```python
from build123d import *

# Parameters (mm, degrees)
F0_W     = 4.7515250481
F0_H     = 22.4042496848
F1_DEPTH = 4.445


with BuildPart() as f1:
    # F0 (on Front) → F1 (new body)
    with BuildSketch(Plane.XZ):
        with BuildLine():
            Line((-107.0503221856, -3.0948602284), (-76.2880815111, 0))
            Line((-76.2880815111, 0), (-86.7243445437, 103.7341952324))
            Line((-86.7243445437, 103.7341952324), (-53.7250275092, 57.9696269721))
            ThreePointArc((-53.7250275092, 57.9696269721), (-46.1566377564, 60.2633619864), (-38.773926276, 57.4283461196))
            Line((-38.773926276, 57.4283461196), (0, 103.7341952324))
            Line((0, 103.7341952324), (40.0807997492, 57.3092244379))
            ThreePointArc((40.0807997492, 57.3092244379), (47.3933296143, 60.2539299742), (54.9783525161, 58.1064171563))
            Line((54.9783525161, 58.1064171563), (86.548257701, 103.7341875683))
            Line((86.548257701, 103.7341875683), (76.1119184889, 0))
            Line((76.1119184889, 0), (106.8741568907, -3.0948828193))
            Line((106.8741568907, -3.0948828193), (148.2956194489, 138.5004273575))
            Line((148.2956194489, 138.5004273575), (-148.4725865748, 138.5004273575))
            Line((-148.4725865748, 138.5004273575), (-107.0503221856, -3.0948602284))
        make_face()
        Polygon((-45.5729805496, 127.6698307823), (-45.5729805496, 109.2178300023), (-50.3245055976, 109.2178300023), (-50.3245055976, 127.6698307823), (-56.4097920627, 127.6698307823), (-56.4097920627, 131.6220796871), (-39.4925976191, 131.6220796871), (-39.4925976191, 127.6698307823), align=None, mode=Mode.SUBTRACT)
        with Locations((-33.6696502563, 120.4199548447)):
            Rectangle(F0_W, F0_H, mode=Mode.SUBTRACT)
        Polygon((-11.0520968155, 113.1406576994), (-11.0520968155, 109.2178300023), (-27.724114528, 109.2178300023), (-27.724114528, 112.2972497445), (-16.9804701727, 127.69925199), (-27.4299024507, 127.69925199), (-27.4299024507, 131.6220796871), (-11.3414053582, 131.6220796871), (-11.3414053582, 128.5573705488), (-22.0703391096, 113.1406576994), align=None, mode=Mode.SUBTRACT)
        Polygon((7.120402491, 113.1406576994), (7.120402491, 109.2178300023), (-9.5516152214, 109.2178300023), (-9.5516152214, 112.2972497445), (1.1920291339, 127.69925199), (-9.2574031441, 127.69925199), (-9.2574031441, 131.6220796871), (6.8310939484, 131.6220796871), (6.8310939484, 128.5573705488), (-3.8978398031, 113.1406576994), align=None, mode=Mode.SUBTRACT)
        with Locations((13.0659382194, 120.4199548447)):
            Rectangle(F0_W, F0_H, mode=Mode.SUBTRACT)
        Polygon((34.9185402592, 109.2178300023), (21.0807655579, 109.2178300023), (21.0807655579, 131.6220796871), (25.832290606, 131.6220796871), (25.832290606, 113.1406576994), (34.9185402592, 113.1406576994), align=None, mode=Mode.SUBTRACT)
        Polygon((41.1411256937, 131.6220796871), (45.7847729801, 122.3985310644), (50.4578414742, 131.6220796871), (55.5771316188, 131.6220796871), (48.1433731329, 117.936314559), (48.1433731329, 109.2178300023), (43.4261728272, 109.2178300023), (43.4261728272, 117.7843049857), (35.9924143413, 131.6220796871), align=None, mode=Mode.SUBTRACT)
        with BuildLine():
            Line((-46.5975366533, 48.0849817395), (-53.7250275092, 57.9696269721))
            ThreePointArc((-53.7250275092, 57.9696269721), (-52.1495262693, 37.2368137569), (-34.411177998, 48.0849817395))
            Line((-34.411177998, 48.0849817395), (-46.5975366533, 48.0849817395))
        make_face()
        with BuildLine():
            ThreePointArc((-38.773926276, 57.4283461196), (-46.1566377564, 60.2633619864), (-53.7250275092, 57.9696269721))
            Line((-53.7250275092, 57.9696269721), (-46.5975366533, 48.0849817395))
            Line((-46.5975366533, 48.0849817395), (-38.773926276, 57.4283461196))
        make_face()
        with BuildLine():
            Line((-38.773926276, 57.4283461196), (-46.5975366533, 48.0849817395))
            Line((-46.5975366533, 48.0849817395), (-34.411177998, 48.0849817395))
            ThreePointArc((-34.411177998, 48.0849817395), (-35.555601603, 53.240852919), (-38.773926276, 57.4283461196))
        make_face()
        with BuildLine():
            ThreePointArc((60.230868841, 48.0849817395), (58.838157085, 53.7422358339), (54.9783525161, 58.1064171563))
            Line((54.9783525161, 58.1064171563), (48.0445101857, 48.0849817395))
            Line((48.0445101857, 48.0849817395), (35.8581515305, 48.0849817395))
            ThreePointArc((35.8581515305, 48.0849817395), (48.0445101857, 35.8986230843), (60.230868841, 48.0849817395))
        make_face()
        with BuildLine():
            Line((48.0445101857, 48.0849817395), (54.9783525161, 58.1064171563))
            ThreePointArc((54.9783525161, 58.1064171563), (47.3933296143, 60.2539299742), (40.0807997492, 57.3092244379))
            Line((40.0807997492, 57.3092244379), (48.0445101857, 48.0849817395))
        make_face()
        with BuildLine():
            Line((48.0445101857, 48.0849817395), (40.0807997492, 57.3092244379))
            ThreePointArc((40.0807997492, 57.3092244379), (36.9639874345, 53.1573926884), (35.8581515305, 48.0849817395))
            Line((35.8581515305, 48.0849817395), (48.0445101857, 48.0849817395))
        make_face()
    extrude(amount=F1_DEPTH)


solid = f1.part
```
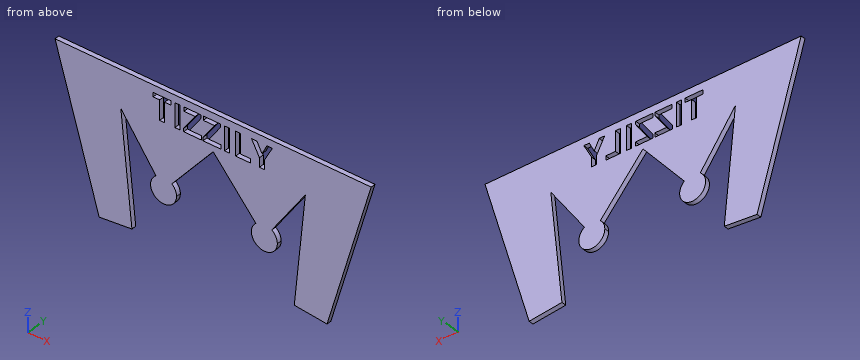
Source: CAD feature listing. Evaluate the final solid. Frame: model axes, mm. Coordinates: 2 decimals unless noted, no trailing zeros. Write each loop counter-clockwise with the first axis right and the second up, starting at its lowest first coordinate (ties: lowest second). Pieces come first, ordered by that corner, then holes. Notation, with made-up numbers: (-24.75, -37.5) - (16.25, -37.5) arc R25 cw to (16.25, -10.5) - close; hole circle Ø2 at (11.25, 78). An arc over 180 degrees is marked (long way). Answer as a JSON object with one key per item and string values.
Q1. Section query B-B, the plane y = -3.05. State how many separate pieces and enclosed holes the cut face has, plus the area to 3 significant figures.
Ans:
{"separate pieces": "1", "enclosed holes": "7", "area": "23,200 mm2"}
Q2. Section query A-A, the plane z = 69.5. Output: boundary loops of the cut face in (x, y) (3 decimals).
Ans:
{"outline": "(-128.287, -4.445) - (-83.28, -4.445) - (-83.28, 0) - (-128.287, 0) - close; (-62.039, -4.445) - (-28.666, -4.445) - (-28.666, 0) - (-62.039, 0) - close; (29.556, -4.445) - (62.862, -4.445) - (62.862, 0) - (29.556, 0) - close; (83.104, -4.445) - (128.111, -4.445) - (128.111, 0) - (83.104, 0) - close"}
Q3. First-contact query: pin 1 Ø2 at (y, z) = (-1.5, 123.5) entering from +X; pin 2 Ø1.2 at (y, z) = (-2.5, 112) entering from -X; pin 3 Ø2 at (x, y) = (-35, -1.5) entering from -Z. Flat tips, straight axial feed; report the tip coordinate or a pass-through.
Ans:
{"pin 1": "stops at x = 144.2", "pin 2": "stops at x = -140.9", "pin 3": "stops at z = 42.07"}
Q4. Section query C-C, the plane z = 41. Output: boundary loops of the cut face in (x, y) (3 decimals).
Ans:
{"outline": "(-119.95, -4.445) - (-80.413, -4.445) - (-80.413, 0) - (-119.95, 0) - close; (-56.513, -4.445) - (-36.682, -4.445) - (-36.682, 0) - (-56.513, 0) - close; (38.129, -4.445) - (57.96, -4.445) - (57.96, 0) - (38.129, 0) - close; (80.237, -4.445) - (119.773, -4.445) - (119.773, 0) - (80.237, 0) - close"}
Q5. Material intervals for line 1 (X direction, y = -0.7, z = 37.5); line 2 (Z direction, x = -12, y = -2.9); line 3 (X direction, y = -1.85, z = 70), sorted ascending. Write a range as [from, to].
Ans:
{"line 1": "x = [-118.93, -80.06], [-52.64, -40.56], [42.01, 54.08], [79.88, 118.75]", "line 2": "z = [89.4, 109.22], [113.14, 127.61], [131.62, 138.5]", "line 3": "x = [-128.43, -83.33], [-62.4, -28.25], [29.12, 63.21], [83.15, 128.26]"}
Q6. Section query D-D, the plane x = -72. Output: boundary loops of the cut face in (y, z) (3 decimals), plus the area to 3 significant figures.
Ans:
{"outline": "(-4.445, 83.314) - (0, 83.314) - (0, 138.5) - (-4.445, 138.5) - close", "area": "245 mm2"}
